The listing builds one solid part. Answer for the finished solid, in the listing's coordinates (mm). A direction names the side the tool comes from. Round coordinates to 2 decimals unless told otherwise and drop trailing zeros. Write each loop counter-clockwise with the first axis right and the second up, starting at its lowest first coordinate (ties: lowest second). Pieces come first, ordered by that corner, then holes. Notation, with made-up numbers: (-28.75, 28) - (5.25, 28) arc R20 ccw to (5.25, 59) - close; hole circle Ø9 at (-29.5, 23). An arc over 180 degrees is marked (long way). Answer as CSV lines item,"result". Start each with the question number.
Item 1: A cutting plane is placed at A-A on y = 0. Determine the outline of the cut face in (x, z), and give its area (3 significant figures).
Item 2: Which of the six approach directions +Z, -Z, +X, -X, +Y, -Y give full straight-line access (tool end or side, diameter ignored) to faces 1 (the flat face through (0, 0, -140)), 2 (the cylindrical face through (-9, 0, -44))?
Item 3: A cutting plane is placed at B-B on x = 0. Determine the outline of the cut face in (y, z).
Item 4: For a pull along Y with two mould halves and no side action, classify faces 3 (the flat face through (-9, 11, -66)), 4 (the cylindrical face through (-12.932, -5.362, -102.504)), 5 (the flat face through (0, 0, -90)) as pulls with the +Y half, pulls with the -Y half, needs draft (parallel to the pull), parting line crosses it, or undercut.
Item 5: Flat-ended cylindrical pins translate along their axes: pin 1 (6 mm diameter, centred on y = 10, z = -54, fed in from +X); pin 2 (1 mm diameter, centred on x = 11, y = -12, fed in from +Z); pin 3 (6 mm diameter, centred on x = 4.5, y = -3.5, fed in from +Z); pin 4 (4 mm diameter, centred on y = -9.5, z = -93, fed in from +X). Find the tip coordinate at first contact, or state that the pin passes through.
Item 6: A cutting plane is placed at D-D on z = -61.5. Determine the outline of the cut face in (x, y).
Item 7: Straight lines are drawn through the part: line 1 along Z through (x, y) = (0, -9.5); line 2 along Y through (x, z) = (0, -39); line 3 along Z through (x, y) = (8, 15). For each, find the intervals that lie inside material, in ascending order. Write a range as [from, to].
Item 8: A cutting plane is placed at C-C on z = -14. Determine the outline of the cut face in (x, y).
Autodesk Inventor part; units mm, degrees
ref_plane "Arbeitsebene1" through (0, 18, 0) normal (0, 1, 0) x (-1, 0, 0)
ref_plane "YZ Plane" through (0, 0, 0) normal (1, 0, 0) x (0, 1, 0)
ref_plane "XY Plane" through (0, 0, 0) normal (0, 0, 1) x (1, 0, 0)
sketch "Skizze1" plane through (0, 0, 0) normal (0, 1, 0) x (-1, 0, 0)
  line L0 (0, 0) -> (18, 0)
  line L1 (18, 0) -> (18, -5)
  line L2 (18, -5) -> (18, -5)
  line L3 (18, -5) -> (18, -11)
  line L4 (18, -11) -> (18, -11)
  line L5 (18, -11) -> (18, -66)
  line L6 (18, -66) -> (14, -66)
  line L7 (14, -66) -> (14, -140)
  line L8 (14, -140) -> (0, -140)
  line L9 (0, -140) -> (0, 0)
  point P0 (18, -8)
  dimension "d0" = 74
  dimension "d1" = 66
  dimension "d5" = 36
  dimension "d6" = 28
revolve "Umdrehung1" add sketch "Skizze1" angle 360 about axis through (0, 0, -140) along (0, 0, 1)
ref_plane "Arbeitsebene1" through (0, 18, 0) normal (0, 1, 0) x (-1, 0, 0)
sketch "Skizze2" plane through (0, 18, 0) normal (0, 1, 0) x (-1, 0, 0)
  point P0 (0, 0)
  point P1 (0, -14)
  dimension "d9" = 14
hole "Bohrung1" at (0, 18, -14) direction (0, -1, 0) diameter 10 end through all
sketch "Skizze3" plane through (0, 0, 0) normal (0, 0, 1) x (1, 0, 0)
  circle A0 centre (0, 0) radius 9
  dimension "d17" = 18
extrude "Extrusion1" cut sketch "Skizze3" against normal blind 90
chamfer "Fasen1" distance 2 angle 45 1 edges at (14, 0, -140)
properties part number "19"
Geometry says:
1,outline,"(-18, -66) - (-14, -66) - (-14, -138) - (-12, -140) - (12, -140) - (14, -138) - (14, -66) - (18, -66) - (18, 0) - (9, 0) - (9, -90) - (-9, -90) - (-9, 0) - (-18, 0) - close"
1,area,"2,820 mm^2"
2,face 1,"-Z, +X, -X, +Y, -Y"
2,face 2,"+Z"
3,outline,"(-18, -66) - (-14, -66) - (-14, -138) - (-12, -140) - (12, -140) - (14, -138) - (14, -66) - (18, -66) - (18, -19) - (9, -19) - (9, -90) - (-9, -90) - (-9, -19) - (-18, -19) - close; (-18, -9) - (-9, -9) - (-9, 0) - (-18, 0) - close; (9, -9) - (18, -9) - (18, 0) - (9, 0) - close"
4,face 3,"needs draft"
4,face 4,"parting line crosses it"
4,face 5,"undercut"
5,pin 1,"stops at x = 16.58"
5,pin 2,"stops at z = 0"
5,pin 3,"stops at z = -90"
5,pin 4,"stops at x = 11.82"
6,outline,"circle Ø36 at (0, 0); hole circle Ø18 at (0, 0)"
7,line 1,"z = [-140, -19], [-9, 0]"
7,line 2,"y = [-18, -9], [9, 18]"
7,line 3,"z = [-66, 0]"
8,outline,"(-5, -17.29) - (-5, -7.48) arc R9 cw to (-5, 7.48) - (-5, 17.29) arc R18 ccw to start; (5, -17.29) arc R18 ccw to (5, 17.29) - (5, 7.48) arc R9 cw to (5, -7.48) - close"
